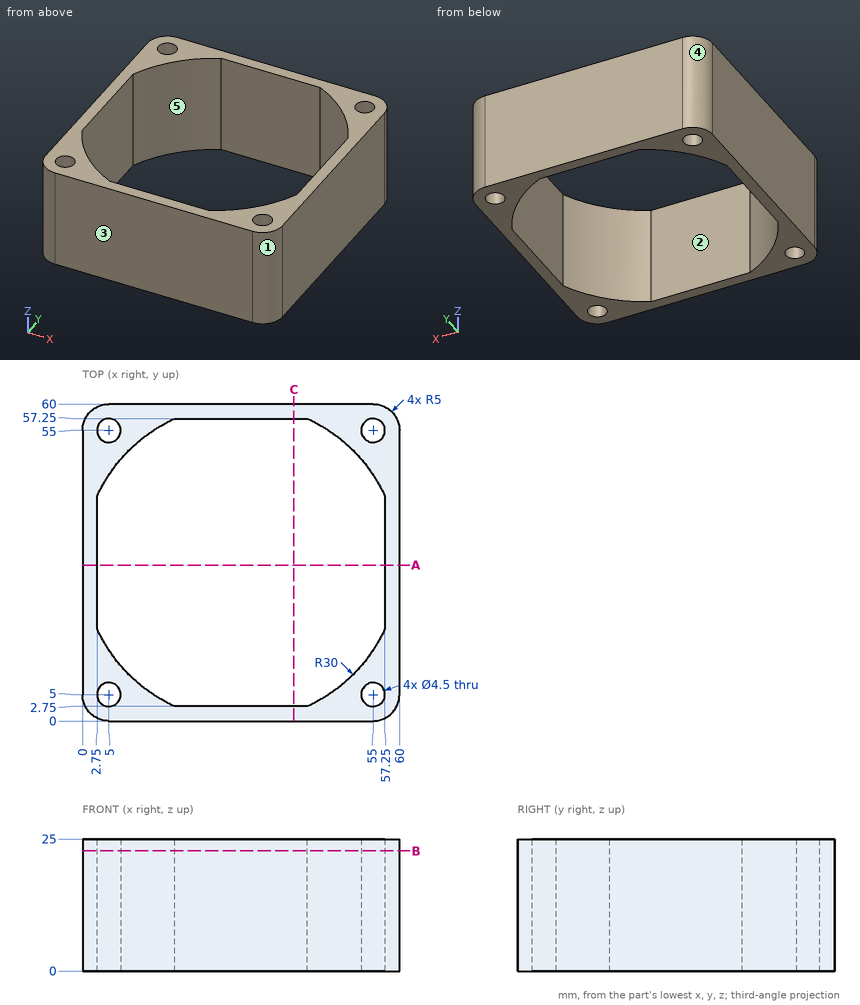
Input: dimensioned drawing with shaded views. Units: mm. Origin: part minimum x, y, z. A direction names the side the tool comes from. Coordinates: 2 decimals unless noted, no trailing zeros. Loops run counter-clockwise (first coordinate to the right, second up) from the corner with the lowest first, then second, coordinate; pieces in that order, holes last. Notation, with made-up numbers: (-13.5, 17) -> (21.5, 17) arc R18 cw to (21.5, 25) -> close; hole circle Ø9 at (60.5, 15.25). An arc over 180 degrees is marked (long way). One line per item, written item: value. Start each with the question number.
Q1. Set-up query: the marked faces 1 and 2. Return all of +Z, -Z, +X, -X, +Y, -Y with unobstructed straight access to the full face (end or side cutting, diameter ignored); none if empty.
Q2. Line query: line 1 along X through (y, z) = (31, 16.75); line 2 along Y through (x, z) = (55, 17.75). Output: solid intervals per line, ascending.
Q3. Section query A-A, the plane y = 29.5. Return the cut outline in (x, z).
Q4. Mould query, pull axis Y, two halves, no side actions, for the marked faces 3, 4 and 5. Classes: pulls with the +Y half, pulls with the -Y half, needs draft (parallel to the pull), parting line crosses it, or undercut.
Q5. Section query B-B, the plane z = 22.75. Return the cut outline in (x, y).
Q6. Contact query for a flat-ended pin moving along its axis: P1, Ø5, axis at x = 55, y = 55, coming from the -Z side. Output: stop coordinate, or through.
Results:
1. face 1: +Z, -Z, +X, -Y
1. face 2: +Z, -Z
2. line 1: 0 to 2.75, 57.25 to 60
2. line 2: 0 to 2.75, 7.25 to 13.42, 46.58 to 52.75, 57.25 to 60
3. outline: (0, 0) -> (2.75, 0) -> (2.75, 25) -> (0, 25) -> close; (57.25, 0) -> (60, 0) -> (60, 25) -> (57.25, 25) -> close
4. face 3: pulls with the -Y half
4. face 4: pulls with the +Y half
4. face 5: undercut
5. outline: (0, 5) arc R5 ccw to (5, 0) -> (55, 0) arc R5 ccw to (60, 5) -> (60, 55) arc R5 ccw to (55, 60) -> (5, 60) arc R5 ccw to (0, 55) -> close; hole circle Ø4.5 at (5, 5); hole (2.75, 17.45) arc R30 ccw to (17.45, 2.75) -> (42.55, 2.75) arc R30 ccw to (57.25, 17.45) -> (57.25, 42.55) arc R30 ccw to (42.55, 57.25) -> (17.45, 57.25) arc R30 ccw to (2.75, 42.55) -> close; hole circle Ø4.5 at (5, 55); hole circle Ø4.5 at (55, 5); hole circle Ø4.5 at (55, 55)
6. P1: z = 0
